For this review, use the dimensioned drawing (mm, ordinates from the lowest corner) and the shaded views. A direction names the side the tool comes from. Round coordinates to 2 decimals unless told otherwise and drop trailing zeros. Loops run counter-clockwise (first coordinate to the right, second up) from the corner with the lowest first, then second, coordinate; pieces in that order, holes last. Notation, with made-up numbers: (89.5, 88) -> (99.5, 88) arc R30 cw to (99.5, 117) -> close; hole circle Ø4 at (-0.75, 42.5). An arc over 180 degrees is marked (long way). Write each question's results on one line, items separated by ' | '.
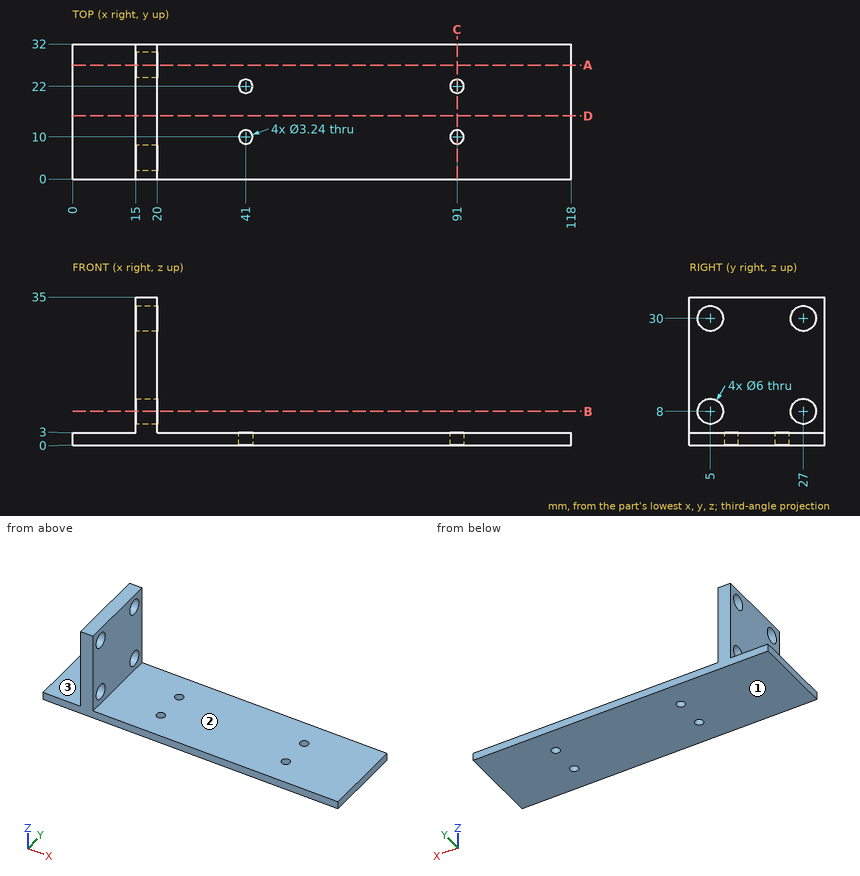
1. Tool access review of the marked faces 1, 2 and 3: name each direction out of +Z, -Z, +X, -X, +Y, -Y from which nothing blocks a thin tool from reaching the whole face with its end or side.
Values found:
face 1: -Z, +X, -X, +Y, -Y | face 2: +Z, +X, +Y, -Y | face 3: +Z, -X, +Y, -Y
2. To check wall thickness, follow probe 1 along Y at (x, z) = (41, 0.9); probe 2 along X at (y, z) = (22, 22); probe 3 along Z at (x, y) = (30, 18). State the ranges of each line that lie inside material, in increasing order.
Values found:
probe 1: y = 0 to 8.38, 11.62 to 20.38, 23.62 to 32 | probe 2: x = 15 to 20 | probe 3: z = 0 to 3
3. Consider section B-B (z = 8). State the section outline as (x, y) points, plus the area to 3 significant figures.
Values found:
outline: (15, 0) -> (20, 0) -> (20, 2) -> (15, 2) -> close; (15, 8) -> (20, 8) -> (20, 24) -> (15, 24) -> close; (15, 30) -> (20, 30) -> (20, 32) -> (15, 32) -> close | area: 100 mm2
4. Consider section D-D (y = 15). State the section outline as (x, z) points.
Values found:
outline: (0, 0) -> (118, 0) -> (118, 3) -> (20, 3) -> (20, 35) -> (15, 35) -> (15, 3) -> (0, 3) -> close
5. For pin 1 (3 mm diameter, centred on y = 19.5, z = 29.5, fed in from -X); pin 2 (2 mm diameter, centred on x = 42, y = 12.5, fed in from +Z); pin 3 (7 mm diameter, centred on y = 5, z = 8, fed in from +X), all flat-tipped, find the tip position at first contact; note any pin that passes through.
Values found:
pin 1: stops at x = 15 | pin 2: stops at z = 3 | pin 3: stops at x = 20
6. Consider section A-A (y = 27). State the section outline as (x, z) points.
Values found:
outline: (0, 0) -> (118, 0) -> (118, 3) -> (20, 3) -> (20, 5) -> (15, 5) -> (15, 3) -> (0, 3) -> close; (15, 11) -> (20, 11) -> (20, 27) -> (15, 27) -> close; (15, 33) -> (20, 33) -> (20, 35) -> (15, 35) -> close
7. Consider section C-C (x = 91). State the section outline as (y, z) points, plus the area to 3 significant figures.
Values found:
outline: (0, 0) -> (8.38, 0) -> (8.38, 3) -> (0, 3) -> close; (11.62, 0) -> (20.38, 0) -> (20.38, 3) -> (11.62, 3) -> close; (23.62, 0) -> (32, 0) -> (32, 3) -> (23.62, 3) -> close | area: 76.6 mm2
